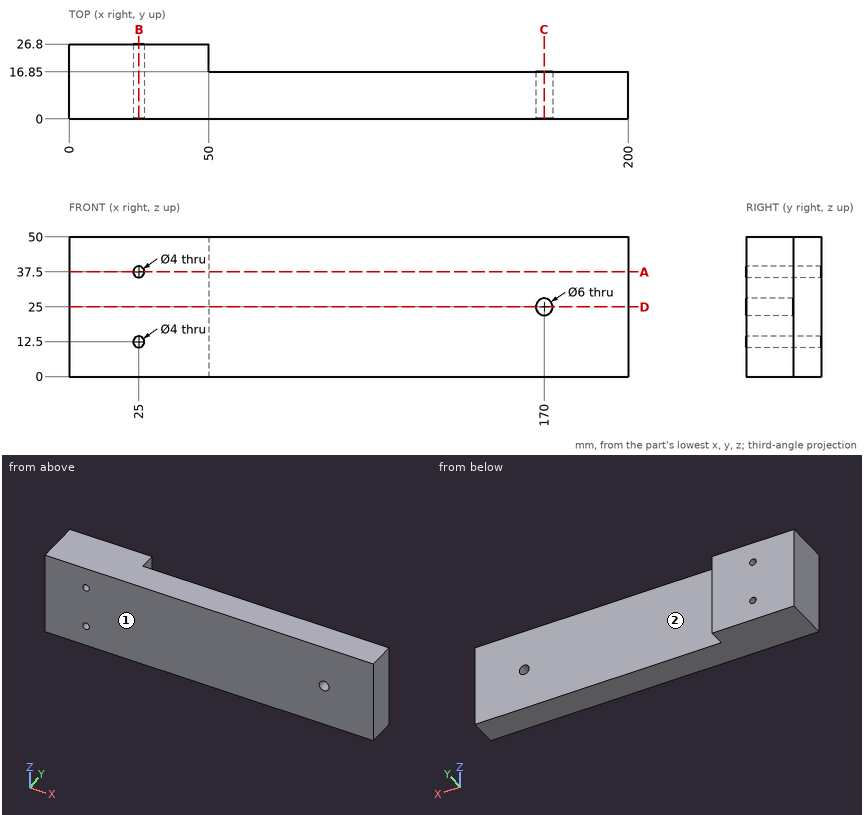
Input: dimensioned drawing with shaded views. Units: mm. Origin: part minimum x, y, z. A direction names the side the tool comes from. Give positions to 0.01 mm unless a question says otherwise; leave off trailing zeros. Write each loop counter-clockwise with the first axis right and the second up, starting at its lowest first coordinate (ties: lowest second). Pieces come first, ordered by that corner, then holes. Notation, with made-up numbers: (12, 60.25) -> (71, 60.25) arc R21 ccw to (71, 80.25) -> close; hole circle Ø2 at (-33, 27). An arc over 180 degrees is marked (long way). Answer as a JSON object with one key per item and string values.
1. Cut plane D-D on z = 25. Output: boundary loops of the cut face in (x, y).
Ans:
{"outline": "(0, 0) -> (167, 0) -> (167, 16.85) -> (50, 16.85) -> (50, 26.8) -> (0, 26.8) -> close; (173, 0) -> (200, 0) -> (200, 16.85) -> (173, 16.85) -> close"}
2. Contact query for flat-ended pins moving along their axis: pin 1 (2 mm diameter, centred on y = 19, z = 7.5, fed in from +X); pin 2 (5 mm diameter, centred on x = 57.5, z = 25.5, fed in from +Y). Output: stop coordinate, or through.
Ans:
{"pin 1": "stops at x = 50", "pin 2": "stops at y = 16.85"}
3. Access query for the marked faces 1 and 2. Directions: +Z, -Z, +X, -X, +Y, -Y. A direction counts if a zero-diameter tool reaches every point of the face in a straight line with its end or side. Return the directions, or none.
Ans:
{"face 1": "+Z, -Z, +X, -X, -Y", "face 2": "+Z, -Z, +X, +Y"}
4. Cut plane B-B on x = 25. Output: boundary loops of the cut face in (y, z), and give its area (3 significant figures).
Ans:
{"outline": "(0, 0) -> (26.8, 0) -> (26.8, 10.5) -> (0, 10.5) -> close; (0, 14.5) -> (26.8, 14.5) -> (26.8, 35.5) -> (0, 35.5) -> close; (0, 39.5) -> (26.8, 39.5) -> (26.8, 50) -> (0, 50) -> close", "area": "1,130 mm^2"}
5. Ray query, probe 1 along X at (y, z) = (12.5, 25); probe 2 along X at (y, z) = (14.75, 37.5); probe 3 along X at (y, z) = (19.5, 40). Return the intervals inside material, ascending. Write a range as from..to.
Ans:
{"probe 1": "x = 0..167, 173..200", "probe 2": "x = 0..23, 27..200", "probe 3": "x = 0..50"}
6. Cut plane C-C on x = 170. Output: boundary loops of the cut face in (y, z), and give its area (3 significant figures).
Ans:
{"outline": "(0, 0) -> (16.85, 0) -> (16.85, 22) -> (0, 22) -> close; (0, 28) -> (16.85, 28) -> (16.85, 50) -> (0, 50) -> close", "area": "741 mm^2"}
7. Cut plane A-A on z = 37.5. Output: boundary loops of the cut face in (x, y).
Ans:
{"outline": "(0, 0) -> (23, 0) -> (23, 26.8) -> (0, 26.8) -> close; (27, 0) -> (200, 0) -> (200, 16.85) -> (50, 16.85) -> (50, 26.8) -> (27, 26.8) -> close"}
